from build123d import *

# Parameters (mm, degrees)
SKETCH_2_W               = 123.4
SKETCH_2_H               = 210
EXTRUDE_2_DEPTH          = 3
EXTRUDE_5_DEPTH          = 4
EXTRUDE_START            = -4
EXTRUDE_6_DEPTH          = 4
EXTRUDE_8_DEPTH          = 8
CUT_EXTRUDE_1_DEPTH      = 205
CUT_EXTRUDE_1_DEPTH_BACK = 243.711170942
SKETCH_8_R               = 2.5
FILLET_1_R               = 3
SKETCH_10_W              = 4
SKETCH_10_H              = 202
EXTRUDE_9_DEPTH          = 45
CUT_EXTRUDE_2_DEPTH      = 182.404830421
SKETCH_12_W              = 3
SKETCH_12_H              = 20
EXTRUDE_10_DEPTH         = 10
CUT_EXTRUDE_3_REACH      = 254.984
SKETCH_13_W              = 99.4
SKETCH_13_H              = 144.727282118
SKETCH_13_W_2            = 205.501958082
SKETCH_13_H_2            = 63.361365512


with BuildPart() as part:
    # 草圖2 → 填料-伸長2 (new body)
    with BuildSketch(Plane.XY):
        with Locations((2.95, -15)):
            Rectangle(SKETCH_2_W, SKETCH_2_H)
    extrude(amount=EXTRUDE_2_DEPTH)

    # 草圖4 → 填料-伸長5 (add)
    with BuildSketch(Plane.XZ.offset(120)):
        with BuildLine():
            Line((-58.75, 3), (-58.75, 58))
            ThreePointArc((-58.75, 58), (2.95, 119.7), (64.65, 58))
            Line((64.65, 58), (64.65, 3))
            Line((64.65, 3), (-58.75, 3))
        make_face()
    extrude(amount=-EXTRUDE_5_DEPTH)

    # 草圖5 → 填料-伸長6 (add)
    with BuildSketch(Plane(origin=(0, 90, 0), x_dir=(1, 0, 0), z_dir=(0, 1, 0)).offset(EXTRUDE_START)):
        with BuildLine():
            Line((-58.75, -3), (-58.75, -58))
            ThreePointArc((-58.75, -58), (2.95, -119.7), (64.65, -58))
            Line((64.65, -58), (64.65, -3))
            Line((64.65, -3), (-58.75, -3))
        make_face()
    extrude(amount=EXTRUDE_6_DEPTH)

    # 草圖7 → 填料-伸長8 (add)
    with BuildSketch(Plane.ZY.offset(58.75)):
        Polygon((3, 86), (58, 86), (58, 81), (48, 81), (48, -111), (58, -111), (58, -116), (3, -116), align=None)
    extrude(amount=-EXTRUDE_8_DEPTH)

    # 草圖8 → 除料-伸長1 (cut, two sides: drawn at the far end of the back side and taken through both)
    with BuildSketch(Plane.XZ.offset(-81).offset(-CUT_EXTRUDE_1_DEPTH_BACK)):
        with Locations(Location((-54.75, 53, 0), (0, 0, 90))):
            Circle(SKETCH_8_R)
    extrude(amount=CUT_EXTRUDE_1_DEPTH + CUT_EXTRUDE_1_DEPTH_BACK, mode=Mode.SUBTRACT)

    # 圓角1
    fillet_1_edges = [part.edges().sort_by_distance(p)[0] for p in [
        (-58.75, -113.5, 58),
        (-58.75, 83.5, 58),
    ]]
    fillet(fillet_1_edges, radius=FILLET_1_R)

    # 草圖10 → 填料-伸長9 (add)
    with BuildSketch(Plane.XY.offset(3)):
        with Locations((62.65, -15)):
            Rectangle(SKETCH_10_W, SKETCH_10_H)
    extrude(amount=EXTRUDE_9_DEPTH)

    # 草圖11 → 除料-伸長2 (cut, through all)
    with BuildSketch(Plane(origin=(0, 0, 0), x_dir=(-1, 0, 0), z_dir=(0, 0, -1))):
        with BuildLine():
            Line((-0.2, -6.75), (-0.2, -23.25))
            ThreePointArc((-0.2, -23.25), (-2.95, -26), (-5.7, -23.25))
            Line((-5.7, -23.25), (-5.7, -6.75))
            ThreePointArc((-5.7, -6.75), (-2.95, -4), (-0.2, -6.75))
        make_face()
    extrude(amount=-CUT_EXTRUDE_2_DEPTH, mode=Mode.SUBTRACT)

    # 草圖12 → 填料-伸長10 (add)
    with BuildSketch(Plane(origin=(64.65, 0, 0), x_dir=(0, 0, -1), z_dir=(1, 0, 0))):
        with Locations((-46.5, -15)):
            Rectangle(SKETCH_12_W, SKETCH_12_H)
    extrude(amount=EXTRUDE_10_DEPTH)

    # 除料-伸長3: up to this face of the body (flat: up to its plane)
    cut_extrude_3_end = Plane(part.part.faces().sort_by_distance((3.036368919, -120, 54.121907078))[0])
    # 草圖13 → 除料-伸長3 (cut, up to the picked face)
    with BuildSketch(Plane(origin=(0, 90, 0), x_dir=(1, 0, 0), z_dir=(0, 1, 0)), mode=Mode.PRIVATE) as cut_extrude_3_sk1:
        with Locations((2.95, -75.363641059)):
            Rectangle(SKETCH_13_W, SKETCH_13_H)
    cut_extrude_3_tool1 = split(extrude(cut_extrude_3_sk1.sketch, amount=-CUT_EXTRUDE_3_REACH, mode=Mode.PRIVATE), bisect_by=cut_extrude_3_end, keep=Keep.BOTH, mode=Mode.PRIVATE)
    # 草圖13 → 除料-伸長3 (cut, up to the picked face)
    with BuildSketch(Plane(origin=(0, 90, 0), x_dir=(1, 0, 0), z_dir=(0, 1, 0)), mode=Mode.PRIVATE) as cut_extrude_3_sk2:
        with Locations((2.95, -89.680682756)):
            Rectangle(SKETCH_13_W_2, SKETCH_13_H_2)
    cut_extrude_3_tool2 = split(extrude(cut_extrude_3_sk2.sketch, amount=-CUT_EXTRUDE_3_REACH, mode=Mode.PRIVATE), bisect_by=cut_extrude_3_end, keep=Keep.BOTH, mode=Mode.PRIVATE)
    add(cut_extrude_3_tool1.solids().sort_by(Axis((2.95, 90, 75.363641), (0, -1, 0)))[0], mode=Mode.SUBTRACT)
    add(cut_extrude_3_tool2.solids().sort_by(Axis((2.95, 90, 89.680683), (0, -1, 0)))[0], mode=Mode.SUBTRACT)


solid = part.part
Could you check a few things on this model? Use its own coordinates, in mm. A direction names the side the tool comes from. Coordinates: 2 decimals unless noted, no trailing zeros. Order: outer loops, then holes, each group sorted by start corner. A loop starts at its lowest first (then second) coordinate and runs counter-clockwise, first axis right, second up. Notation, with made-up numbers: (86, 19) - (93, 19) arc R19 cw to (93, 48) - close; hole circle Ø7 at (60, 86). An arc over 180 degrees is marked (long way). Answer in a Markdown table with one row per item. Add a question column.
(1) On a 3-axis mill with a long thin cutter (end or side, diameter ignored), from which of +Z, -Z, +X, -X, +Y, -Y can I reach the whole of each face in a straight line? I mean faces 4 (the face through (70, -15, 45)), 5 (the face through (52.65, -118, 31)), 6 (the face through (-52, 81, 53)). Say none if no direction works.
(2) Will these pins go through, and if not, where does the flat tip stop? pin 1 (2 mm diameter, centred on y = 89, z = 42.5, fed in from +X); pin 2 (15.5 mm diameter, centred on x = 65.5, y = 12.5, fed in from +Z); pin 3 (12 mm diameter, centred on x = 46.5, z = 15, fed in from +Y) (3 decimals); pin 4 (2 mm diameter, centred on x = -44.5, y = 15.5, fed in from +Z).
(3) If we section it at D-D, the plane x = 55.5: Please give me the cut outline in (y, z), then the cut area to 3 significant figures.
(4) If we section it at C-C, the plane y = -46.5: Please give me the cut outline in (x, z), then the cut area to 3 significant figures.
(5) If we mould it in two halves opening along X, with no side actions, what happens to faces 1 (the face through (-53, -116, 58)), 2 (the face through (-58.75, -14, 23)), 3 (the face through (-46.75, 88, 31))? For each: released by +X, released by -X, zero draft, split by the parting line, or undercut.
(6) If we section it at B-B, the plane x = 2.95: Please give me the cut outline in (y, z).
(7) I need wall thicknesses on L1, parallel to X at y = -116.5, z = 53; L2, parallel to X at y = 5, z = 33; L3, parallel to X at y = -114, z = 53. Which ranges of each line are inside material? Lowest first, please.
(8) If we section it at A-A, the plane z = 20.5: Please give me the cut outline in (x, y).
Results are:
| question | item | result |
|---|---|---|
| 1 | face 4 | -Z, +X, +Y, -Y |
| 1 | face 5 | +Z, +Y, -Y |
| 1 | face 6 | +Z, +X, -X |
| 2 | pin 1 | stops at x = 64.65 |
| 2 | pin 2 | stops at z = 48 |
| 2 | pin 3 | passes through |
| 2 | pin 4 | stops at z = 3 |
| 3 | outline | (-120, 0) - (90, 0) - (90, 58) - (86, 58) - (86, 3) - (-116, 3) - (-116, 58) - (-120, 58) - close |
| 3 | area | 1,070 mm2 |
| 4 | outline | (-58.75, 0) - (64.65, 0) - (64.65, 48) - (60.65, 48) - (60.65, 3) - (-50.75, 3) - (-50.75, 48) - (-58.75, 48) - close |
| 4 | area | 910 mm2 |
| 5 | face 1 | zero draft |
| 5 | face 2 | released by -X |
| 5 | face 3 | undercut |
| 6 | outline | (-120, 0) - (-26, 0) - (-26, 3) - (-120, 3) - close; (-4, 0) - (90, 0) - (90, 3) - (-4, 3) - close |
| 7 | L1 | x = -58.75 to -57.25, -52.25 to -46.75, 52.65 to 64.65 |
| 7 | L2 | x = -58.75 to -50.75, 60.65 to 64.65 |
| 7 | L3 | x = -58.75 to -57.25, -52.25 to -50.75 |
| 8 | outline | (-58.75, -120) - (-46.75, -120) - (-46.75, -116) - (-50.75, -116) - (-50.75, 86) - (-46.75, 86) - (-46.75, 90) - (-58.75, 90) - close; (52.65, -120) - (64.65, -120) - (64.65, 90) - (52.65, 90) - (52.65, 86) - (60.65, 86) - (60.65, -116) - (52.65, -116) - close |
